Verification items for the finished model (mm, model axes). A direction names the side the tool comes from. Coordinates: 2 decimals unless noted, no trailing zeros. Order: outer loops, then holes, each group sorted by start corner. A loop starts at its lowest first (then second) coordinate and runs counter-clockwise, first axis right, second up. Notation, with made-up numbers: M 14,27 L 49,27 A19 ccw 49,32 Z; hole C -4,30.25 d6. An arc over 180 degrees is marked long. Return JSON: item names as keys, results as strings.
```python
from build123d import *

# Parameters (mm, degrees)
EXTRUDE_1_DEPTH     = 2
SKETCH_2_W          = 1
SKETCH_2_H          = 8
EXTRUDE_2_DEPTH     = 9
FILLET_2_R          = 3
SKETCH_3_R          = 1.5
CUT_EXTRUDE_1_DEPTH = 20


with BuildPart() as part:
    # 草图1 → 凸台-拉伸1 (new body)
    with BuildSketch(Plane(origin=(0, 0, 0), x_dir=(1, 0, 0), z_dir=(0, 1, 0))):
        with BuildLine():
            Line((-16, 4), (16, 4))
            ThreePointArc((16, 4), (17.414213562, 3.414213562), (18, 2))
            Line((18, 2), (18, -2))
            ThreePointArc((18, -2), (17.414213562, -3.414213562), (16, -4))
            Line((16, -4), (-16, -4))
            ThreePointArc((-16, -4), (-17.414213562, -3.414213562), (-18, -2))
            Line((-18, -2), (-18, 2))
            ThreePointArc((-18, 2), (-17.414213562, 3.414213562), (-16, 4))
        make_face()
        with BuildLine():
            Line((-9, -1.5), (-15, -1.5))
            ThreePointArc((-15, -1.5), (-16.5, 0), (-15, 1.5))
            Line((-15, 1.5), (-9, 1.5))
            ThreePointArc((-9, 1.5), (-7.5, 0), (-9, -1.5))
        make_face(mode=Mode.SUBTRACT)
        with BuildLine():
            Line((9, 1.5), (15, 1.5))
            ThreePointArc((15, 1.5), (16.5, 0), (15, -1.5))
            Line((15, -1.5), (9, -1.5))
            ThreePointArc((9, -1.5), (7.5, 0), (9, 1.5))
        make_face(mode=Mode.SUBTRACT)
    extrude(amount=EXTRUDE_1_DEPTH)

    # 草图2 → 凸台-拉伸2 (add)
    with BuildSketch(Plane(origin=(0, 2, 0), x_dir=(1, 0, 0), z_dir=(0, 1, 0))):
        with Locations((4.5, 0)):
            Rectangle(SKETCH_2_W, SKETCH_2_H)
        with Locations((-4.5, 0)):
            Rectangle(SKETCH_2_W, SKETCH_2_H)
    extrude(amount=EXTRUDE_2_DEPTH)

    # 圆角2
    fillet_2_edges = [part.edges().sort_by_distance(p)[0] for p in [
        (4.5, 11, -4),
        (4.5, 11, 4),
        (-4.5, 11, -4),
        (-4.5, 11, 4),
    ]]
    fillet(fillet_2_edges, radius=FILLET_2_R)

    # 草图3 → 切除-拉伸1 (cut)
    with BuildSketch(Plane.ZY.offset(5)):
        with Locations((0, 7)):
            Circle(SKETCH_3_R)
    extrude(amount=-CUT_EXTRUDE_1_DEPTH, mode=Mode.SUBTRACT)


solid = part.part
```
Q1. Go/stop test with flat-tipped pins: pin 1 (3 mm diameter, centred on x = 14.5, y = 4, fed in from -Z); pin 2 (1.5 mm diameter, centred on y = 9.5, z = -2, fed in from +X); pin 3 (5 mm diameter, centred on x = 3, y = 9, fed in from -Z). Record where each tip stops, or that it passes through.
Values:
{"pin 1": "through", "pin 2": "x = 5", "pin 3": "z = -4"}
Q2. Cross-section at C-C, the plane y = 7. Record the boundary of the cut face in (x, z).
Values:
{"outline": "M -5,-4 L -4,-4 L -4,-1.5 L -5,-1.5 Z; M -5,1.5 L -4,1.5 L -4,4 L -5,4 Z; M 4,-4 L 5,-4 L 5,-1.5 L 4,-1.5 Z; M 4,1.5 L 5,1.5 L 5,4 L 4,4 Z"}
Q3. Cross-section at B-B, the plane z = 0. Record the boundary of the cut face in (x, y).
Values:
{"outline": "M -18,0 L -16.5,0 L -16.5,2 L -18,2 Z; M -7.5,0 L 7.5,0 L 7.5,2 L 5,2 L 5,5.5 L 4,5.5 L 4,2 L -4,2 L -4,5.5 L -5,5.5 L -5,2 L -7.5,2 Z; M -5,8.5 L -4,8.5 L -4,11 L -5,11 Z; M 4,8.5 L 5,8.5 L 5,11 L 4,11 Z; M 16.5,0 L 18,0 L 18,2 L 16.5,2 Z"}
Q4. Tool access check on faces 4 (the face through (-4, 5, 0)), 5 (the face through (-5, 5, 0)), 6 (the face through (12, 2, 2)). Record the directions out of +Z, -Z, +X, -X, +Y, -Y that give a thin tool (end or side, any length) a straight path to the whole face; none if there is none.
Values:
{"face 4": "+Z, -Z, +Y", "face 5": "+Z, -Z, -X, +Y", "face 6": "+Z, -Z, +X, +Y"}
Q5. Cross-section at A-A, the plane y = 3.75. Record the boundary of the cut face in (x, z).
Values:
{"outline": "M -5,-4 L -4,-4 L -4,4 L -5,4 Z; M 4,-4 L 5,-4 L 5,4 L 4,4 Z"}
Q6. Cross-section at D-D, the plane y = 9.25. Record the boundary of the cut face in (x, z), and give its area (3 significant figures).
Values:
{"outline": "M -5,-3.73 L -4,-3.73 L -4,3.73 L -5,3.73 Z; M 4,-3.73 L 5,-3.73 L 5,3.73 L 4,3.73 Z", "area": "14.9 mm^2"}
Q7. Draft check along Z on faces 1 (the face through (-4.507, 5.536, -0.325)), 2 (the face through (-18, 1, 0)), 3 (the face through (-4.49, 10.1, 3.14)). Enter one of: pulls with the +Z half, pulls with the -Z half, needs draft (parallel to the pull), parting line crosses it, or undercut.
Values:
{"face 1": "undercut", "face 2": "needs draft", "face 3": "pulls with the +Z half"}
Q8. Material ranges on line 1 along Z through (x, y) = (10, 1.5); line 2 along X through (y, z) = (3.5, -2); line 3 along Y through (x, z) = (-4.2, 0), recorded low to high.
Values:
{"line 1": "-4 to -1.5, 1.5 to 4", "line 2": "-5 to -4, 4 to 5", "line 3": "0 to 5.5, 8.5 to 11"}
